from build123d import *

# Parameters (mm, degrees)
F2_SIZE  = 1
F3_R     = 30
F4_DEPTH = 25
F3_R_2   = 3
F5_DEPTH = 25


with BuildPart() as f1:
    # F0 (on Right) → F1 (revolve)
    with BuildSketch(Plane.YZ):
        Polygon((-19, 7.675), (-19, 6), (10.5, 6), (10.5, 8.9), (9, 8.9), (9, 7), (6, 7), (6, 8.9), (4, 8.9), (4, 24), (0, 24), (0, 7.175), (-16.5, 7.175), (-16.5, 7.675), align=None)
    revolve(axis=Axis((0, -3.653569, 0), (0, 1, 0)))

    # F2
    f2_edges = [f1.edges().sort_by_distance(p)[0] for p in [
        (0, -19, -7.675),
    ]]
    chamfer(f2_edges, length=F2_SIZE)

    # F3 (on face) → F4 (cut)
    with BuildSketch(Plane.XZ):
        Circle(F3_R)
        with BuildLine():
            ThreePointArc((-19.914286, -6.035), (-24, 0), (-19.914286, 6.035))
            Line((-19.914286, 6.035), (-4.828571, 12.07))
            ThreePointArc((-4.828571, 12.07), (0, 13), (4.828571, 12.07))
            Line((4.828571, 12.07), (19.914286, 6.035))
            ThreePointArc((19.914286, 6.035), (24, 0), (19.914286, -6.035))
            Line((19.914286, -6.035), (4.828571, -12.07))
            ThreePointArc((4.828571, -12.07), (0, -13), (-4.828571, -12.07))
            Line((-4.828571, -12.07), (-19.914286, -6.035))
        make_face(mode=Mode.SUBTRACT)
    extrude(amount=-F4_DEPTH, mode=Mode.SUBTRACT)

    # F3 (on face) → F5 (cut)
    with BuildSketch(Plane.XZ):
        with Locations((17.5, 0)):
            Circle(F3_R_2)
        with Locations((-17.5, 0)):
            Circle(F3_R_2)
    extrude(amount=-F5_DEPTH, mode=Mode.SUBTRACT)


solid = f1.part
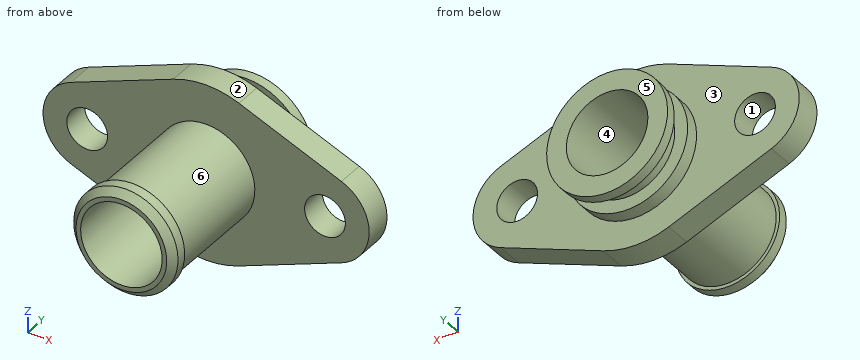
Can you work these out from the model? Positions are in its coordinate system, mm. Face numbers are marked on the shaded views. A direction names the side the tool comes from. Round coordinates to 2 decimals unless told otherwise and drop trailing zeros. Order: outer loops, then holes, each group sorted by start corner. A loop starts at its lowest first (then second) coordinate and runs counter-clockwise, first axis right, second up. Notation, with made-up numbers: (30.5, 29.25) - (48.5, 29.25) arc R14 ccw to (48.5, 37.25) - close; hole circle Ø9 at (27, 76.5). An arc over 180 degrees is marked (long way). Answer in a Markdown table with one row per item.
(1) Suppose I cut it at A-A, the plane y = 1.75. Please give me the cut outline in (x, z) (3 decimals), plus the area to 3 significant figures.
From the geometry:
| item | result |
|---|---|
| outline | (-19.914, -6.035) - (-4.829, -12.07) arc R13 ccw to (4.829, -12.07) - (19.914, -6.035) arc R6.5 ccw to (19.914, 6.035) - (4.829, 12.07) arc R13 ccw to (-4.829, 12.07) - (-19.914, 6.035) arc R6.5 ccw to start; hole circle Ø6 at (-17.5, 0); hole circle Ø12 at (0, 0); hole circle Ø6 at (17.5, 0) |
| area | 693 mm2 |
(2) If we mould it in two halves opening along Z, with no side actions, what happens to the marked faces 1, 2, 3 and 4? For each: released by +Z, released by -Z, zero draft, split by the parting line, or undercut.
From the geometry:
| item | result |
|---|---|
| face 1 | undercut |
| face 2 | released by +Z |
| face 3 | zero draft |
| face 4 | undercut |
(3) Which directions (+Z, -Z, +X, -X, +Y, -Y) give clear straight access to the entire face, cutting with the end or side of a thin tool? Please do the marked faces 5 and 6.
From the geometry:
| item | result |
|---|---|
| face 5 | +Z, -Z, +X, -X, +Y |
| face 6 | none |
(4) Suppose I cut it at D-D, the plane z = 8.25. Please give me the cut outline in (x, y).
From the geometry:
| item | result |
|---|---|
| outline | (-14.38, 0) - (14.38, 0) - (14.38, 4) - (3.34, 4) - (3.34, 6) - (-3.34, 6) - (-3.34, 4) - (-14.38, 4) - close; (-3.34, 9) - (3.34, 9) - (3.34, 10.5) - (-3.34, 10.5) - close |
(5) For P1, Ø4, axis at y = 4.5, z = -5.5, coming from the -X side; P2, Ø8, axis at x = -16.5, z = 3.5, coming from the -Y side; P3, Ø8, axis at x = -0.5, y = -15, coming from the +Z side (3 decimals), each with a flat end and sliding along its axis, tell me the tip position at first contact or that it passes through.
From the geometry:
| item | result |
|---|---|
| P1 | stops at x = -22.94 |
| P2 | stops at y = 0 |
| P3 | stops at z = 7.675 |
(6) Suppose I cut it at C-C, the plane z = 0. Count the separate pieces of the cut face and the enclosed holes in it, plus the area to 3 significant figures.
From the geometry:
| item | result |
|---|---|
| separate pieces | 4 |
| enclosed holes | 0 |
| area | 168 mm2 |
(7) Please list where these lines run through material, in increasing order: L1, parallel to X at y = -5.5, z = 0 (3 decimals); L2, parallel to Y at x = -2.5, z = -8; L3, parallel to Y at x = -11.5, z = -4.75. Write a range as from..to.
From the geometry:
| item | result |
|---|---|
| L1 | x = -7.175..-6, 6..7.175 |
| L2 | y = 0..6, 9..10.5 |
| L3 | y = 0..4 |
